Read the model definition and answer for the solid it produces. Units are mm, in the model's axes. Face numbers are marked on the shaded views. Round coordinates to 2 decimals unless told otherwise and drop trailing zeros. Write each loop counter-clockwise with the first axis right and the second up, starting at its lowest first coordinate (ties: lowest second). Pieces come first, ordered by that corner, then holes.
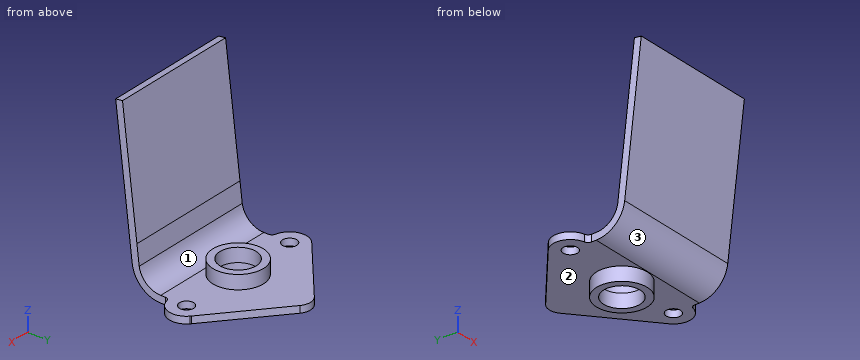
from build123d import *
from build123d.topology import SkipClean

# Parameters (mm, degrees)
SKETCH2_R           = 3.125
SKETCH2_R_2         = 7.9375
BOSS_EXTRUDE2_DEPTH = 3
BOSS_EXTRUDE3_START = 6
SKETCH5_R           = 11
SKETCH5_R_2         = 7.9375
BOSS_EXTRUDE3_DEPTH = 6
SKETCH6_R           = 11
SKETCH6_R_2         = 7.9375
BOSS_EXTRUDE4_DEPTH = 6
BOSS_EXTRUDE5_DEPTH = 56
FILLET1_R           = 2


with BuildPart() as part:
    # Sketch2 → Boss-Extrude2 (new body)
    # profile 1 of 2: a face of its own
    with BuildSketch(Plane.XY):
        with BuildLine():
            ThreePointArc((3.861106297, 30.092587306), (0, 31.5), (-3.861106297, 30.092587306))
            Line((-3.861106297, 30.092587306), (-32.826382871, 5.740734133))
            ThreePointArc((-32.826382871, 5.740734133), (-35.046470961, -2.568510658), (-28, -7.5))
            Line((-28, -7.5), (-28, -11.25))
            Line((-28, -11.25), (28, -11.25))
            Line((28, -11.25), (28, -7.5))
            ThreePointArc((28, -7.5), (35.006811058, -2.674808179), (32.997833475, 5.592106988))
            Line((32.997833475, 5.592106988), (32.651575677, 5.883268116))
            Line((32.651575677, 5.883268116), (3.86193439, 30.091890979))
            Line((3.86193439, 30.091890979), (3.861106297, 30.092587306))
        make_face()
        with Locations((-28, 0)):
            Circle(SKETCH2_R, mode=Mode.SUBTRACT)
        with BuildLine():
            ThreePointArc((0, -11), (-0.700886243, -10.97764813), (-1.3989241, -10.910683359))
            ThreePointArc((-1.3989241, -10.910683359), (-7.266768019, 8.25797085), (11, 0))
            ThreePointArc((11, 0), (7.778174593, -7.778174593), (0, -11))
        make_face(mode=Mode.SUBTRACT)
        with Locations((28, 0)):
            Circle(SKETCH2_R, mode=Mode.SUBTRACT)
    # profile 2 of 2: a face of its own
    with BuildSketch(Plane.XY):
        with BuildLine():
            ThreePointArc((11, 0), (-7.266768019, 8.25797085), (-1.3989241, -10.910683359))
            ThreePointArc((-1.3989241, -10.910683359), (-0.700886243, -10.97764813), (0, -11))
            ThreePointArc((0, -11), (7.778174593, -7.778174593), (11, 0))
        make_face()
        Circle(SKETCH2_R_2, mode=Mode.SUBTRACT)
    extrude(amount=BOSS_EXTRUDE2_DEPTH)

    # Sketch5 → Boss-Extrude3 (add)
    with SkipClean():  # the faces are left unmerged after this step: merging them gives an invalid solid
        with BuildSketch(Plane(origin=(0, 0, 0), x_dir=(-1, 0, 0), z_dir=(0, 0, -1)).offset(BOSS_EXTRUDE3_START)):
            with Locations(Location((0, 0, 0), (0, 0, 180))):
                Circle(SKETCH5_R)
            Circle(SKETCH5_R_2, mode=Mode.SUBTRACT)
        extrude(amount=-BOSS_EXTRUDE3_DEPTH)

    # Sketch6 → Boss-Extrude4 (add)
    with BuildSketch(Plane.XY.offset(3)):
        Circle(SKETCH6_R)
        with Locations(Location((0, 0, 0), (0, 0, 180))):
            Circle(SKETCH6_R_2, mode=Mode.SUBTRACT)
    extrude(amount=BOSS_EXTRUDE4_DEPTH)

    # Sketch8 → Boss-Extrude5 (add)
    with BuildSketch(Plane.ZY.offset(28)):
        with BuildLine():
            Line((73, -27.9), (19.471115904, -21.625622538))
            Line((19.471115904, -21.625622538), (11.046076805, -20.638083262))
            ThreePointArc((11.046076805, -20.638083262), (5.286738936, -17.432140796), (3, -11.25))
            Line((3, -11.25), (0, -11.25))
            ThreePointArc((0, -11.25), (3.161262399, -19.558909677), (11.046076805, -23.665156356))
            Line((11.046076805, -23.665156356), (72.651058433, -30.879637525))
            Line((72.651058433, -30.879637525), (73, -27.9))
        make_face()
    extrude(amount=-BOSS_EXTRUDE5_DEPTH)

    # Fillet1
    fillet1_edges = [part.edges().sort_by_distance(p)[0] for p in [
        (-28, -7.5, 1.5),
        (28, -7.5, 1.5),
    ]]
    fillet(fillet1_edges, radius=FILLET1_R)


solid = part.part
Q1. Straight lines are drawn through the part: probe 1 along Y at (x, z) = (0, 4.6); probe 2 along Y at (x, z) = (0, -4.05); probe 3 along Z at (x, y) = (7, 17.5). For each, find the intervals that lie inside material, in ascending order.
Verdict:
probe 1: y = -20.94 to -16.53, -11 to -7.94, 7.94 to 11
probe 2: y = -11 to -7.94, 7.94 to 11
probe 3: z = 0 to 3
Q2. Flat-ended cylindrical pins translate along their axes: pin 1 Ø8 at (x, z) = (2, 22.5) entering from -Y; pin 2 Ø8 at (x, y) = (-28, 0) entering from -Z; pin 3 Ø11 at (y, z) = (-24, 29.5) entering from -X. Find the tip coordinate at first contact, or state that the pin passes through.
Verdict:
pin 1: stops at y = -25.47
pin 2: stops at z = 0
pin 3: stops at x = -28
Q3. Section A-A (x = 0) is taken. Determine the outline of the cut face in (y, z), then the cut area to 3 significant figures.
Verdict:
outline: (-30.88, 72.65) - (-23.67, 11.05) arc R12.5 ccw to (-11.25, 0) - (-11, 0) - (-11, -6) - (-7.94, -6) - (-7.94, 9) - (-11, 9) - (-11, 3) - (-11.25, 3) arc R9.5 cw to (-20.64, 11.05) - (-27.9, 73) - close; (7.94, -6) - (11, -6) - (11, 0) - (31.5, 0) - (31.5, 3) - (11, 3) - (11, 9) - (7.94, 9) - close
area: 388 mm2
Q4. Section D-D (x = 26) is taken. Determine the outline of the cut face in (y, z).
Verdict:
outline: (-30.88, 72.65) - (-23.67, 11.05) arc R12.5 ccw to (-11.25, 0) - (-2.4, 0) - (-2.4, 3) - (-11.25, 3) arc R9.5 cw to (-20.64, 11.05) - (-27.9, 73) - close; (2.4, 0) - (11.48, 0) - (11.48, 3) - (2.4, 3) - close
Q5. Section B-B (y = 0) is taken. Determine the outline of the cut face in (x, z) (1 decimal), then the cut area to 3 significant figures.
Verdict:
outline: (-35.5, 0) - (-31.1, 0) - (-31.1, 3) - (-35.5, 3) - close; (-24.9, 0) - (-11, 0) - (-11, -6) - (-7.9, -6) - (-7.9, 9) - (-11, 9) - (-11, 3) - (-24.9, 3) - close; (7.9, -6) - (11, -6) - (11, 0) - (24.9, 0) - (24.9, 3) - (11, 3) - (11, 9) - (7.9, 9) - close; (31.1, 0) - (35.5, 0) - (35.5, 3) - (31.1, 3) - close
area: 201 mm2
Q6. Determine the mould class of the marked faces 1, 2 and 3 for opening direction Y: pulls with the +Y half, pulls with the -Y half, needs draft (parallel to the pull), parting line crosses it, or undercut.
Verdict:
face 1: undercut
face 2: needs draft
face 3: pulls with the -Y half
Q7. Section C-C (x = -18) is taken. Determine the outline of the cut face in (y, z).
Verdict:
outline: (-30.88, 72.65) - (-23.67, 11.05) arc R12.5 ccw to (-11.25, 0) - (18.21, 0) - (18.21, 3) - (-11.25, 3) arc R9.5 cw to (-20.64, 11.05) - (-27.9, 73) - close
